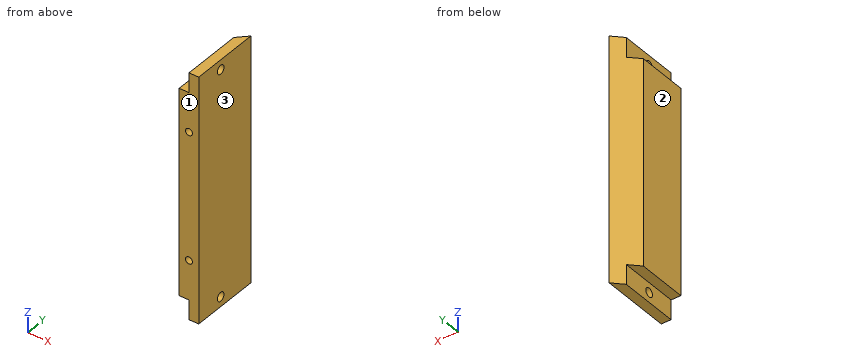
from build123d import *

# Parameters (mm, degrees)
SKETCH1_W                 = 39.6875
SKETCH1_H                 = 22.6314
SKETCH1_R                 = 1.4351
BOSS_EXTRUDE1_DEPTH       = 6.35
SKETCH2_W                 = 3.175
SKETCH2_H                 = 6.35
CUT_EXTRUDE1_DEPTH        = 47.125919202
CUT_EXTRUDE2_DEPTH        = 47.125919202
F_4_40_TAPPED_HOLE1_D     = 2.2606
F_4_40_TAPPED_HOLE1_DEPTH = 9.652
F_4_40_TAPPED_HOLE1_TIP   = 0.679152758


with BuildPart() as part:
    # Sketch1 → Boss-Extrude1 (new body)
    with BuildSketch(Plane(origin=(0, 0, 0), x_dir=(0, 0, -1), z_dir=(1, 0, 0))):
        with Locations((19.84375, 11.3157)):
            Rectangle(SKETCH1_W, SKETCH1_H)
        with Locations((36.5125, 9.525)):
            Circle(SKETCH1_R, mode=Mode.SUBTRACT)
    extrude(amount=-BOSS_EXTRUDE1_DEPTH)

    # Sketch2 → Cut-Extrude1 (cut, through all)
    with BuildSketch(Plane.XZ):
        with Locations((-4.7625, -36.5125)):
            Rectangle(SKETCH2_W, SKETCH2_H)
    extrude(amount=-CUT_EXTRUDE1_DEPTH, mode=Mode.SUBTRACT)

    # Sketch3 → Cut-Extrude2 (cut, through all)
    with BuildSketch(Plane.XY):
        Polygon((0, 22.6314), (-6.35, 16.2814), (-6.35, 22.6314), align=None)
    extrude(amount=-CUT_EXTRUDE2_DEPTH, mode=Mode.SUBTRACT)

    # #4-40 Tapped Hole1
    with Locations(Plane.XZ):
        with Locations((-3.175, -20.6375)):
            Hole(F_4_40_TAPPED_HOLE1_D / 2, depth=F_4_40_TAPPED_HOLE1_DEPTH)
            with Locations((0, 0, -(F_4_40_TAPPED_HOLE1_DEPTH + F_4_40_TAPPED_HOLE1_TIP / 2))):  # 118° drill point
                Cone(0, F_4_40_TAPPED_HOLE1_D / 2, F_4_40_TAPPED_HOLE1_TIP, mode=Mode.SUBTRACT)

    # Mirror1: part across plane


with BuildPart() as part_1:
    add(part.part)
    add(part.part.mirror(Plane(origin=(-6.35, 0, 0), x_dir=(1, 0, 0), z_dir=(0, 0, 1))))


solid = part_1.part
The listing builds one solid part. Answer for the finished solid, in the listing's coordinates (mm). Face numbers are marked on the shaded views. Coordinates: 2 decimals unless noted, no trailing zeros. Loops run counter-clockwise (first coordinate to the right, second up) from the corner with the lowest first, then second, coordinate; pieces in that order, holes last. Notation, with made-up numbers: M 86,56.25 L 140,56.25 A23 cw 140,88.25 Z; hole C -32,-15 d8. An arc over 180 degrees is marked long. Answer in a Markdown table with one row per item.
1) Find section B-B (y = 6.75). Count the separate pieces of the cut face and the enclosed holes in it, then the cut area to 3 significant figures.
Answers below:
| item | result |
|---|---|
| separate pieces | 1 |
| enclosed holes | 2 |
| area | 456 mm^2 |
2) Find section C-C (z = -34). Determine the outline of the cut face in (x, y) (3 decimals), then the cut area to 3 significant figures.
Answers below:
| item | result |
|---|---|
| outline | M -3.175,0 L 0,0 L 0,22.631 L -3.175,19.456 Z |
| area | 66.8 mm^2 |
3) Given pin 1 (2.5 mm diameter, centred on y = 9.52, z = -36.51, fed in from -X); pin 2 (1 mm diameter, centred on x = -4.5, y = 11, fed in from -Z); pin 3 (2.5 mm diameter, centred on x = -3.18, z = 20.64, fed in from +Y); pin 4 (2 mm diameter, centred on x = -5.5, z = -7.5, fed in from +Y), each flat-ended and moving along its own axis, determine where each tip first touches the part or whether it passes through.
Answers below:
| item | result |
|---|---|
| pin 1 | through |
| pin 2 | z = -33.34 |
| pin 3 | y = 20.7 |
| pin 4 | y = 18.13 |
4) Determine the mould class of the marked faces 1, 2 and 3 for opening direction X: released by +X, released by -X, zero draft, split by the parting line, or undercut.
Answers below:
| item | result |
|---|---|
| face 1 | zero draft |
| face 2 | released by -X |
| face 3 | released by +X |
5) Find the intervals of material crossed by probe 1 along Z at (x, y) = (-3.5, 3.75); probe 2 along Z at (x, y) = (-4, 3.5); probe 3 along Z at (x, y) = (-6, 13), in increasing order.
Answers below:
| item | result |
|---|---|
| probe 1 | -33.34 to -21.72, -19.55 to 19.55, 21.72 to 33.34 |
| probe 2 | -33.34 to -21.41, -19.86 to 19.86, 21.41 to 33.34 |
| probe 3 | -33.34 to 33.34 |
6) Find section D-D (x = -1.25). Determine the outline of the cut face in (y, z) (1 decimal), then the cut area to 3 significant figures.
Answers below:
| item | result |
|---|---|
| outline | M 0,-39.7 L 21.4,-39.7 L 21.4,39.7 L 0,39.7 Z; hole C 9.5,-36.5 d2.9; hole C 9.5,36.5 d2.9 |
| area | 1,680 mm^2 |
